Could you check a few things on this model? Use its own coordinates, in mm. A direction names the side the tool comes from. Give positions to 0.01 mm unless a question says otherwise; leave off trailing zeros. Loops run counter-clockwise (first coordinate to the right, second up) from the corner with the lowest first, then second, coordinate; pieces in that order, holes last. Notation, with made-up numbers: (49.25, -20) - (54.25, -20) arc R10 cw to (54.25, -9) - close; hole circle Ø4 at (80.25, 10.5). An arc over 180 degrees is marked (long way). Answer in a Markdown table with one row per item. Add a question column.
```python
from build123d import *

# Parameters (mm, degrees)
SKETCH_1_W      = 7
SKETCH_1_H      = 4
EXTRUDE_1_DEPTH = 0.6
SKETCH_2_W      = 5.8
SKETCH_2_H      = 2.8
EXTRUDE_2_DEPTH = 2.2
FILLET_1_R      = 1
SKETCH_3_W      = 3
SKETCH_3_H      = 1.6
EXTRUDE_3_DEPTH = 0.1
FILLET_2_R      = 0.2


with BuildPart() as part:
    # 草图1 → 凸台-拉伸1 (new body)
    with BuildSketch(Plane(origin=(0, 0, 0), x_dir=(1, 0, 0), z_dir=(0, 1, 0))):
        with Locations((0.996893044, -0.239645207)):
            Rectangle(SKETCH_1_W, SKETCH_1_H)
    extrude(amount=EXTRUDE_1_DEPTH)

    # 草图2 → 凸台-拉伸2 (add)
    with BuildSketch(Plane(origin=(0, 0.6, 0), x_dir=(1, 0, 0), z_dir=(0, 1, 0))):
        with Locations((0.996893044, -0.239645207)):
            Rectangle(SKETCH_2_W, SKETCH_2_H)
    extrude(amount=EXTRUDE_2_DEPTH)

    # 圆角1
    fillet_1_edges = [part.edges().sort_by_distance(p)[0] for p in [
        (3.896893044, 1.7, 1.639645207),
        (3.896893044, 1.7, -1.160354793),
        (-1.903106956, 1.7, -1.160354793),
        (-1.903106956, 1.7, 1.639645207),
        (-2.503106956, 0.3, -1.760354793),
        (4.496893044, 0.3, -1.760354793),
        (4.496893044, 0.3, 2.239645207),
        (-2.503106956, 0.3, 2.239645207),
    ]]
    fillet(fillet_1_edges, radius=FILLET_1_R)

    # 草图3 → 凸台-拉伸3 (add)
    with BuildSketch(Plane(origin=(0, 0, 0), x_dir=(-1, 0, 0), z_dir=(0, -1, 0))):
        with Locations((-0.996893044, -0.239645207)):
            Rectangle(SKETCH_3_W, SKETCH_3_H)
    extrude(amount=EXTRUDE_3_DEPTH)

    # 圆角2
    fillet_2_edges = [part.edges().sort_by_distance(p)[0] for p in [
        (0.996893044, 2.8, -1.160354793),
        (3.896893044, 2.8, 0.239645207),
        (-1.903106956, 2.8, 0.239645207),
        (0.996893044, 2.8, 1.639645207),
        (3.603999825, 2.8, 1.346751988),
        (-1.610213737, 2.8, 1.346751988),
        (-1.610213737, 2.8, -0.867461574),
        (3.603999825, 2.8, -0.867461574),
    ]]
    fillet(fillet_2_edges, radius=FILLET_2_R)


solid = part.part
```
(1) I want a section at B-B on y = 0.9. Please give me the cut outline in (x, z), then the cut area to 3 significant figures.
(2) For pin 1 Ø1 at (x, z) = (-1.5, -1) entering from -Y, with a flat end and sliding along its axis, tell me the tip position at first contact or that it passes through.
(3) Please list where these lines run through material, in increasing order: line 1 (Y direction, x = -1.75, z = 1.5); line 2 (Z direction, x = 0, y = 1.05); line 3 (Y direction, x = 0, z = 1.1).
(4) I want a section at A-A on x = 0. Please give me the cut outline in (y, z), then the cut area to 3 significant figures.
(5) On a 3-axis mill with a long thin cutter (end or side, diameter ignored), from which of +Z, -Z, +X, -X, +Y, -Y can I reach the whole of each face in a straight line? I mean faces 1 (the flat face through (1, 2, -1.16)), 2 (the cylindrical face through (3.61, 1.61, -0.86)), 3 (the flat face through (-1.903, 2, 0)). Say none if no direction works.
(6) I want a section at D-D on x = -2. Please give me the cut outline in (y, z), then the cut area to 3 significant figures.
(7) I want a section at C-C on y = 0.2. Please give me the cut outline in (x, z).
Reported:
| question | item | result |
|---|---|---|
| 1 | outline | (-1.9, -0.16) arc R1 ccw to (-0.9, -1.16) - (2.9, -1.16) arc R1 ccw to (3.9, -0.16) - (3.9, 0.64) arc R1 ccw to (2.9, 1.64) - (-0.9, 1.64) arc R1 ccw to (-1.9, 0.64) - close |
| 1 | area | 15.4 mm² |
| 2 | pin 1 | y = 0 |
| 3 | line 1 | 0 to 0.6 |
| 3 | line 2 | -1.16 to 1.64 |
| 3 | line 3 | 0 to 2.8 |
| 4 | outline | (-0.1, -0.56) - (0, -0.56) - (0, -1.76) - (0.6, -1.76) - (0.6, -1.16) - (2.6, -1.16) arc R0.2 ccw to (2.8, -0.96) - (2.8, 1.44) arc R0.2 ccw to (2.6, 1.64) - (0.6, 1.64) - (0.6, 2.24) - (0, 2.24) - (0, 1.04) - (-0.1, 1.04) - close |
| 4 | area | 8.70 mm² |
| 5 | face 1 | -Z, +X, -X, +Y |
| 5 | face 2 | -Z, +X, +Y |
| 5 | face 3 | +Z, -Z, -X, +Y |
| 6 | outline | (0, -1.63) - (0.6, -1.63) - (0.6, 2.11) - (0, 2.11) - close |
| 6 | area | 2.24 mm² |
| 7 | outline | (-2.5, -0.76) arc R1 ccw to (-1.5, -1.76) - (3.5, -1.76) arc R1 ccw to (4.5, -0.76) - (4.5, 1.24) arc R1 ccw to (3.5, 2.24) - (-1.5, 2.24) arc R1 ccw to (-2.5, 1.24) - close |
